```python
from build123d import *

# Parameters (mm, degrees)
F0_W     = 35
F0_H     = 15
F1_DEPTH = 60
F2_DEPTH = 40
F3_DEPTH = 40


with BuildPart() as f1:
    # F0 (on Front) → F1 (new body)
    with BuildSketch(Plane.XZ):
        Polygon((-20, 0), (0, 0), (0, 30), (-20, 30), (-20, 15), align=None)
        Polygon((-20, 30), (0, 30), (0, 45), (-55, 45), (-55, 35), (-20, 35), align=None)
        with Locations((-37.5, 7.5)):
            Rectangle(F0_W, F0_H)
    extrude(amount=-F1_DEPTH)

    # F0 (on Front) → F2 (cut)
    with BuildSketch(Plane.XZ):
        Polygon((-20, 30), (0, 30), (0, 45), (-55, 45), (-55, 35), (-20, 35), align=None)
    extrude(amount=-F2_DEPTH, mode=Mode.SUBTRACT)

    # F0 (on Front) → F3 (cut)
    with BuildSketch(Plane.XZ):
        with Locations((-37.5, 7.5)):
            Rectangle(F0_W, F0_H)
    extrude(amount=-F3_DEPTH, mode=Mode.SUBTRACT)


solid = f1.part
```
Part model, mm, in its own coordinate system. A direction names the side the tool comes from. Coordinates: 2 decimals unless noted, no trailing zeros. Loops run counter-clockwise (first coordinate to the right, second up) from the corner with the lowest first, then second, coordinate; pieces in that order, holes last. Notation, with made-up numbers: (78, -23.5) - (135, -23.5) arc R16 cw to (135, -19.5) - close; hole circle Ø10 at (89.25, 64.5). An arc over 180 degrees is marked (long way). Write item = value, one per line. Start each with the question number.
Item 1: Cut at C-C, the plane z = 6. Give the cut face in (x, y).
Item 2: 3-axis set-ups, long thin cutter, end or side, ignore diameter. For faces 4 (the flat face through (0, 30, 17)), 5 (the flat face through (-38, 50, 35)), 6 (the flat face through (-38, 40, 8)), 7 (the flat face through (-28, 40, 39)): which of +Z, -Z, +X, -X, +Y, -Y reach the whole face in a straight line?
Item 3: Cut at D-D, the plane x = -17. Give the cut face in (y, z).
Item 4: Cut at A-A, the plane x = -43. Give the cut face in (y, z), and give its area (3 significant figures).
Item 5: Flat gauge pins, fed straight in: pin 1 Ø6 at (x, z) = (-45, 7.5) entering from -Y; pin 2 Ø6 at (y, z) = (22, 8) entering from -X; pin 3 Ø6 at (y, z) = (11.5, 33.5) entering from -X; pin 4 Ø10 at (x, y) = (-15, 23.5) entering from +Z. Where does each tip first touch, or does it go through?
Item 6: Mould opens along Z. For faces 1 (the flat face through (-38, 50, 15)), 2 (the flat face through (-16, 60, 23)), 3 (the flat face through (-27, 50, 45)) say: released by +Z, released by -Z, zero draft, split by the parting line, or undercut.
Item 7: Cut at B-B, the plane y = 49. Give the cut face in (x, z).
Item 8: Wall check: L1, parallel to Z at x = -25, y = 45; L2, parallel to X at y = 41, z = 26.5; L3, parallel to Y at x = -26.5, z = 38. Give the ranges that are in metal, low to high. Write a range as from..to.
The answers:
q1.outline = (-55, 40) - (-20, 40) - (-20, 0) - (0, 0) - (0, 60) - (-55, 60) - close
q2.face_4 = +Z, -Z, +X, +Y, -Y
q2.face_5 = -X, +Y, -Y
q2.face_6 = +Z, -Z, -X, -Y
q2.face_7 = +Z, +X, -X, -Y
q3.outline = (0, 0) - (60, 0) - (60, 45) - (40, 45) - (40, 30) - (0, 30) - close
q4.outline = (40, 0) - (60, 0) - (60, 15) - (40, 15) - close; (40, 35) - (60, 35) - (60, 45) - (40, 45) - close
q4.area = 500 mm2
q5.pin_1 = 40
q5.pin_2 = -20
q5.pin_3 = through
q5.pin_4 = 30
q6.face_1 = undercut
q6.face_2 = zero draft
q6.face_3 = released by +Z
q7.outline = (-55, 0) - (0, 0) - (0, 45) - (-55, 45) - (-55, 35) - (-20, 35) - (-20, 15) - (-55, 15) - close
q8.L1 = 0..15, 35..45
q8.L2 = -20..0
q8.L3 = 40..60
